from build123d import *

# Parameters (mm, degrees)
SKETCH_1_W                          = 50
SKETCH_1_H                          = 255
EXTRUDE_1_DEPTH                     = 10
SKETCH_2_W                          = 50
SKETCH_2_H                          = 9
CUT_EXTRUDE_1_DEPTH                 = 1
PATTERN_LINEAR_1_COUNT              = 5
PATTERN_LINEAR_1_PITCH              = 60
HOLE_WIZARD_M3_1_D                  = 3.4
HOLE_WIZARD_M3_1_CBORE_D            = 6.5
HOLE_WIZARD_M3_1_CBORE_DEPTH        = 3
PATTERN_LINEAR_2_COUNT              = 2
PATTERN_LINEAR_2_PITCH              = 15
PATTERN_LINEAR_3_COUNT              = 2
PATTERN_LINEAR_3_PITCH              = 120
PATTERN_LINEAR_3_COPY_1_D           = 3.4
PATTERN_LINEAR_3_COPY_1_CBORE_D     = 6.5
PATTERN_LINEAR_3_COPY_1_CBORE_DEPTH = 3
PATTERN_LINEAR_4_COUNT              = 2
PATTERN_LINEAR_4_PITCH              = 20
PATTERN_LINEAR_4_COPY_1_D           = 3.4
PATTERN_LINEAR_4_COPY_1_CBORE_D     = 6.5
PATTERN_LINEAR_4_COPY_1_CBORE_DEPTH = 3
PATTERN_LINEAR_4_COPY_2_D           = 3.4
PATTERN_LINEAR_4_COPY_2_CBORE_D     = 6.5
PATTERN_LINEAR_4_COPY_2_CBORE_DEPTH = 3
PATTERN_LINEAR_4_COPY_3_D           = 3.4
PATTERN_LINEAR_4_COPY_3_CBORE_D     = 6.5
PATTERN_LINEAR_4_COPY_3_CBORE_DEPTH = 3
SKETCH_6_W                          = 27
SKETCH_6_H                          = 2
CUT_EXTRUDE_2_DEPTH                 = 138.318061449
PATTERN_LINEAR_5_COUNT              = 2
PATTERN_LINEAR_5_PITCH              = 120
CUT_EXTRUDE_3_DEPTH                 = 131.312125299
CHAMFER_1_SIZE                      = 2
HOLE_WIZARD_M3_1_2_D                = 2.5
SKETCH_10_R                         = 2
CUT_EXTRUDE_4_DEPTH                 = 131.312125299


with BuildPart() as part:
    # Sketch 1 → Extrude 1 (new body)
    with BuildSketch(Plane(origin=(0, 0, 0), x_dir=(1, 0, 0), z_dir=(0, 1, 0))):
        Rectangle(SKETCH_1_W, SKETCH_1_H)
    extrude(amount=EXTRUDE_1_DEPTH)

    # Sketch 2 → Cut-Extrude 1 (cut)
    with BuildSketch(Plane(origin=(0, 10, 0), x_dir=(1, 0, 0), z_dir=(0, 1, 0))):
        with Locations((0, -120)):
            Rectangle(SKETCH_2_W, SKETCH_2_H)
        with Locations((0, -102.4)):
            Rectangle(SKETCH_2_W, SKETCH_2_H)
    cut_extrude_1 = extrude(amount=-CUT_EXTRUDE_1_DEPTH, mode=Mode.SUBTRACT)

    # Pattern Linear 1: Cut-Extrude 1 ×5
    with Locations(*[(0, 0, -i * PATTERN_LINEAR_1_PITCH) for i in range(1, PATTERN_LINEAR_1_COUNT)]):
        add(cut_extrude_1, mode=Mode.SUBTRACT)

    # Hole Wizard M3 _1 (through all)
    with Locations(Plane(origin=(0, 10, 0), x_dir=(-1, 0, 0), z_dir=(0, 1, 0))):
        with Locations((5.5, 51.2)):
            hole_wizard_m3_1 = CounterBoreHole(HOLE_WIZARD_M3_1_D / 2, HOLE_WIZARD_M3_1_CBORE_D / 2, HOLE_WIZARD_M3_1_CBORE_DEPTH)

    # Pattern Linear 2: Hole Wizard M3 _1 ×2
    with Locations(*[(i * PATTERN_LINEAR_2_PITCH, 0, 0) for i in range(1, PATTERN_LINEAR_2_COUNT)]):
        add(hole_wizard_m3_1, mode=Mode.SUBTRACT)

    # Pattern Linear 3: Hole Wizard M3 _1 ×2
    with Locations(*[(0, 0, -i * PATTERN_LINEAR_3_PITCH) for i in range(1, PATTERN_LINEAR_3_COUNT)]):
        add(hole_wizard_m3_1, mode=Mode.SUBTRACT)

    # Pattern Linear 3 copy 1 (through all)
    with Locations(Plane(origin=(15, 10, -120), x_dir=(-1, 0, 0), z_dir=(0, 1, 0))):
        with Locations((5.5, 51.2)):
            CounterBoreHole(PATTERN_LINEAR_3_COPY_1_D / 2, PATTERN_LINEAR_3_COPY_1_CBORE_D / 2, PATTERN_LINEAR_3_COPY_1_CBORE_DEPTH)

    # Pattern Linear 4: Hole Wizard M3 _1 ×2
    with Locations(*[(0, 0, i * PATTERN_LINEAR_4_PITCH) for i in range(1, PATTERN_LINEAR_4_COUNT)]):
        add(hole_wizard_m3_1, mode=Mode.SUBTRACT)

    # Pattern Linear 4 copy 1 (through all)
    with Locations(Plane(origin=(15, 10, 20), x_dir=(-1, 0, 0), z_dir=(0, 1, 0))):
        with Locations((5.5, 51.2)):
            CounterBoreHole(PATTERN_LINEAR_4_COPY_1_D / 2, PATTERN_LINEAR_4_COPY_1_CBORE_D / 2, PATTERN_LINEAR_4_COPY_1_CBORE_DEPTH)

    # Pattern Linear 4 copy 2 (through all)
    with Locations(Plane(origin=(0, 10, -100), x_dir=(-1, 0, 0), z_dir=(0, 1, 0))):
        with Locations((5.5, 51.2)):
            CounterBoreHole(PATTERN_LINEAR_4_COPY_2_D / 2, PATTERN_LINEAR_4_COPY_2_CBORE_D / 2, PATTERN_LINEAR_4_COPY_2_CBORE_DEPTH)

    # Pattern Linear 4 copy 3 (through all)
    with Locations(Plane(origin=(15, 10, -100), x_dir=(-1, 0, 0), z_dir=(0, 1, 0))):
        with Locations((5.5, 51.2)):
            CounterBoreHole(PATTERN_LINEAR_4_COPY_3_D / 2, PATTERN_LINEAR_4_COPY_3_CBORE_D / 2, PATTERN_LINEAR_4_COPY_3_CBORE_DEPTH)

    # Sketch 6 → Cut-Extrude 2 (cut, through all)
    with BuildSketch(Plane(origin=(25, 0, 0), x_dir=(0, 0, -1), z_dir=(1, 0, 0))):
        with Locations((-61.2, 1)):
            Rectangle(SKETCH_6_W, SKETCH_6_H)
    cut_extrude_2 = extrude(amount=-CUT_EXTRUDE_2_DEPTH, mode=Mode.SUBTRACT)

    # Pattern Linear 5: Cut-Extrude 2 ×2
    with Locations(*[(0, 0, -i * PATTERN_LINEAR_5_PITCH) for i in range(1, PATTERN_LINEAR_5_COUNT)]):
        add(cut_extrude_2, mode=Mode.SUBTRACT)

    # Sketch 7 → Cut-Extrude 3 (cut, through all)
    with BuildSketch(Plane(origin=(0, 10, 0), x_dir=(1, 0, 0), z_dir=(0, 1, 0))):
        with BuildLine():
            Line((25, -5.5), (22.2, -5.5))
            Line((22.2, -5.5), (22.2, -8))
            ThreePointArc((22.2, -8), (22.053553391, -8.353553391), (21.7, -8.5))
            Line((21.7, -8.5), (18.2, -8.5))
            ThreePointArc((18.2, -8.5), (17.846446609, -8.353553391), (17.7, -8))
            Line((17.7, -8), (17.7, 8))
            ThreePointArc((17.7, 8), (17.846446609, 8.353553391), (18.2, 8.5))
            Line((18.2, 8.5), (21.7, 8.5))
            ThreePointArc((21.7, 8.5), (22.053553391, 8.353553391), (22.2, 8))
            Line((22.2, 8), (22.2, 5.5))
            Line((22.2, 5.5), (25, 5.5))
            Line((25, 5.5), (25, -5.5))
        make_face()
    extrude(amount=-CUT_EXTRUDE_3_DEPTH, mode=Mode.SUBTRACT)

    # Chamfer 1
    chamfer_1_edges = [part.edges().sort_by_distance(p)[0] for p in [
        (25, 5, 127.5),
        (-25, 5, 127.5),
        (-25, 5, -127.5),
        (25, 5, -127.5),
    ]]
    chamfer(chamfer_1_edges, length=CHAMFER_1_SIZE)

    # Hole Wizard M3 _1 2 (through all)
    with Locations(Plane(origin=(0, 10, 0), x_dir=(-1, 0, 0), z_dir=(0, 1, 0))):
        with Locations((17.5, 120.75), (17.5, 102.15), (2.5, 120.75), (2.5, 102.15), (17.5, 60.75), (2.5, 60.75), (2.5, 42.15), (17.5, 42.15), (17.5, 0.75), (2.5, 0.75), (2.5, -17.85), (17.5, -17.85), (17.5, -59.25), (2.5, -59.25), (2.5, -77.85), (17.5, -77.85), (17.5, -120.75), (2.5, -120.75)):
            Hole(HOLE_WIZARD_M3_1_2_D / 2)

    # Sketch 10 → Cut-Extrude 4 (cut, through all)
    with BuildSketch(Plane(origin=(0, 10, 0), x_dir=(1, 0, 0), z_dir=(0, 1, 0))):
        with Locations(Location((7, 120, 0), (0, 0, 270))):
            Circle(SKETCH_10_R)
        with Locations(Location((7, 77.6, 0), (0, 0, 270))):
            Circle(SKETCH_10_R)
        with Locations(Location((7, 60, 0), (0, 0, 270))):
            Circle(SKETCH_10_R)
        with Locations(Location((7, 17.6, 0), (0, 0, 270))):
            Circle(SKETCH_10_R)
        with Locations(Location((7, 0, 0), (0, 0, 270))):
            Circle(SKETCH_10_R)
        with Locations(Location((7, -42.4, 0), (0, 0, 270))):
            Circle(SKETCH_10_R)
        with Locations(Location((7, -60, 0), (0, 0, 270))):
            Circle(SKETCH_10_R)
        with Locations(Location((7, -102.4, 0), (0, 0, 270))):
            Circle(SKETCH_10_R)
        with Locations(Location((7, -120, 0), (0, 0, 270))):
            Circle(SKETCH_10_R)
    extrude(amount=-CUT_EXTRUDE_4_DEPTH, mode=Mode.SUBTRACT)


solid = part.part
CAD build for the part. Positions are in the model's coordinates, mm. A direction names the side the tool comes from. Coordinates: 2 decimals unless noted, no trailing zeros. Use a Markdown table: item, result. Add a question column.
Item 1: 3-axis set-ups, long thin cutter, end or side, ignore diameter. For faces 1 (the face through (17.7, 5, 0)), 2 (the face through (0, 2, -59)), 3 (the face through (-7, 7, -70)): which of +Z, -Z, +X, -X, +Y, -Y reach the whole face in a straight line?
Item 2: Drill centre lines: L1, parallel to X at y = 3.7, z = -68.8; L2, parallel to Z at x = 13, y = 1.75; L3, parallel to Z at x = 9.5, y = 5.25. Where is each one in solid material? Low to high. Write a range as from..to.
Item 3: Flat gauge pins, fed straight in: pin 1 (1.5 mm diameter, centred on x = -2.5, z = 42.15, fed in from +Y); pin 2 (3 mm diameter, centred on x = -17.5, z = 60.75, fed in from +Y). Where does each tip first touch, or does it go through?
Item 4: Mould opens along Z. For faces 4 (the face through (0, 0, -100)), 5 (the face through (-5.077, 8.521, -65.578)), 6 (the face through (0, 9, 60)) say: pulls with the +Z half, pulls with the -Z half, needs draft (parallel to the pull), parting line crosses it, or undercut.
Numbers:
| question | item | result |
|---|---|---|
| 1 | face 1 | +Y, -Y |
| 1 | face 2 | +X, -X, -Y |
| 1 | face 3 | +Y |
| 2 | L1 | -25..-7.2, -3.8..7.8, 11.2..25 |
| 2 | L2 | -127.5..-72.3, -45.3..47.7, 74.7..127.5 |
| 2 | L3 | -127.5..-70.5, -67.1..-50.5, -47.1..49.5, 52.9..69.5, 72.9..127.5 |
| 3 | pin 1 | through |
| 3 | pin 2 | y = 9 |
| 4 | face 4 | needs draft |
| 4 | face 5 | undercut |
| 4 | face 6 | undercut |
